Source: CAD feature listing. Evaluate the final solid. Frame: model axes, mm. Give positions to 0.01 mm unless a question says otherwise; leave off trailing zeros. Order: outer loops, then holes, each group sorted by start corner. A loop starts at its lowest first (then second) coordinate and runs counter-clockwise, first axis right, second up. Notation, with made-up numbers: M -19.75,69.5 L 16.25,69.5 A4 cw 16.25,73.5 Z; hole C -28.75,33.5 d8. An arc over 180 degrees is marked long. Return JSON: item names as keys, results as strings.
from build123d import *

# Parameters (mm, degrees)
SKETCH1_W                = 12.8
SKETCH1_H                = 14
BOSS_EXTRUDE1_DEPTH      = 6.5
FILLET1_R                = 1
BOSS_EXTRUDE2_DEPTH      = 0.2
BOSS_EXTRUDE2_DEPTH_BACK = 3


with BuildPart() as part:
    # Sketch1 → Boss-Extrude1 (new body)
    with BuildSketch(Plane(origin=(0, 0, 0), x_dir=(1, 0, 0), z_dir=(0, 1, 0))):
        with Locations((6.4, 7)):
            Rectangle(SKETCH1_W, SKETCH1_H)
    extrude(amount=BOSS_EXTRUDE1_DEPTH)

    # Fillet1
    fillet1_edges = [part.edges().sort_by_distance(p)[0] for p in [
        (0, 3.25, 0),
        (0, 3.25, -14),
        (12.8, 3.25, -14),
        (12.8, 3.25, 0),
    ]]
    fillet(fillet1_edges, radius=FILLET1_R)

    # Sketch2 → Boss-Extrude2 (add, two sides: drawn at the far end of the back side and taken through both)
    with BuildSketch(Plane.XZ.offset(-BOSS_EXTRUDE2_DEPTH_BACK)):
        Polygon((8.9, 0), (8.9, -2.6), (3.9, -2.6), (3.9, 0.5), (8.9, 0.5), align=None)
        Polygon((3.9, -14.5), (8.9, -14.5), (8.9, -14), (8.9, -11.4), (3.9, -11.4), align=None)
    extrude(amount=BOSS_EXTRUDE2_DEPTH + BOSS_EXTRUDE2_DEPTH_BACK)


solid = part.part
1. Section query D-D (y = 0.75). Return loops of the section in (x, z), then the cut area to 3 significant figures.
Evaluation:
{"outline": "M 0,-13 A1 ccw 1,-14 L 3.9,-14 L 3.9,-14.5 L 8.9,-14.5 L 8.9,-14 L 11.8,-14 A1 ccw 12.8,-13 L 12.8,-1 A1 ccw 11.8,0 L 8.9,0 L 8.9,0.5 L 3.9,0.5 L 3.9,0 L 1,0 A1 ccw 0,-1 Z", "area": "183 mm^2"}
2. Draft query along Z for faces 1 (the face through (6, 6.5, -7)), 2 (the face through (6, 0, -7)), 3 (the face through (12.499, 3.296, -0.285)). Return one class per face: pulls with the +Z half, pulls with the -Z half, needs draft (parallel to the pull), parting line crosses it, or undercut.
Evaluation:
{"face 1": "needs draft", "face 2": "undercut", "face 3": "pulls with the +Z half"}
3. Section query B-B (x = 6.25). Return loops of the section in (y, z), then the cut area to 3 significant figures.
Evaluation:
{"outline": "M -0.2,-14.5 L 3,-14.5 L 3,-14 L 6.5,-14 L 6.5,0 L 3,0 L 3,0.5 L -0.2,0.5 L -0.2,-2.6 L 0,-2.6 L 0,-11.4 L -0.2,-11.4 Z", "area": "95.2 mm^2"}
4. Section query A-A (z = -12). Return loops of the section in (x, y), then the cut area to 3 significant figures.
Evaluation:
{"outline": "M 0,0 L 3.9,0 L 3.9,-0.2 L 8.9,-0.2 L 8.9,0 L 12.8,0 L 12.8,6.5 L 0,6.5 Z", "area": "84.2 mm^2"}
5. Section query C-C (y = 4.5). Return loops of the section in (x, z).
Evaluation:
{"outline": "M 0,-13 A1 ccw 1,-14 L 11.8,-14 A1 ccw 12.8,-13 L 12.8,-1 A1 ccw 11.8,0 L 1,0 A1 ccw 0,-1 Z"}
6. Ray query, probe 1 along Y at (x, z) = (5.5, -6.25); probe 2 along Z at (x, y) = (1.5, 0.75); probe 3 along X at (y, z) = (2.25, -13.5). Return the intervals inside material, ascending.
Evaluation:
{"probe 1": "y = 0 to 6.5", "probe 2": "z = -14 to 0", "probe 3": "x = 0.13 to 12.67"}
